Check sheet for the modelled part. Datum: model origin and axes. Units: mm. A direction names the side the tool comes from. Coordinates: 2 decimals unless noted, no trailing zeros. Loops run counter-clockwise (first coordinate to the right, second up) from the corner with the lowest first, then second, coordinate; pieces in that order, holes last. Notation, with made-up numbers: (-35, 82.5) - (-14, 82.5) arc R22 cw to (-14, 91.5) - close; hole circle Ø3 at (79, -30). An arc over 180 degrees is marked (long way). Write each question's results on one line, items separated by ' | '. Start each with the question number.
1. Cross-section at A-A (z = 0). Record the cut outline in (x, y).
2. Draft check along Z on faces 1 (the face through (-27.1, 31.1, -15.4)), 2 (the face through (27.937, 51.549, 15.191)), 3 (the face through (30.092, 33.799, -20.509)). Enter one of: released by +Z, released by -Z, zero draft, split by the parting line, or undercut.
3. Cross-section at B-B (y = 36.75). Record the cut outline in (x, z).
4. Thickness scan on line 1 (Z direction, x = 0, y = 51.45); line 2 (Z direction, x = 0, y = 53.75); line 3 (X direction, y = 52, z = 16). Record the ranges inside material, lowest first. Write a range as [from, to].
5. Gauge pin test, flat ends, axial feed: P1, Ø1, axis at y = 32.5, z = 36.5, coming from the -X side; P2, Ø1.8, axis at x = 25.49, z = 13.83, coming from the -Y side; P3, Ø12, axis at y = 35.5, z = -0.5, coming from the -X side; P4, Ø4, axis at x = -8.5, y = 50.5, coming from the +Z side. Record the tip position at first contact, or that the pin passes through.
6. Tool access check on faces 4 (the face through (32.8, 33.8, -15.8)), 5 (the face through (31, 34.1, -19)), 6 (the face through (-29.95, 32.086, -20.756)). Record the directions out of +Z, -Z, +X, -X, +Y, -Y that give a thin tool (end or side, any length) a straight path to the whole face; none if there is none.
```python
from build123d import *

# Parameters (mm, degrees)
SKETCH1_R                = 35
SKETCH1_R_2              = 2.6
SKETCH1_R_3              = 11
BOSS_EXTRUDE1_DEPTH      = 50
SKETCH2_R                = 31
CUT_EXTRUDE1_DEPTH       = 45
SKETCH3_R                = 26.05
SKETCH3_R_2              = 23.55
BOSS_EXTRUDE2_DEPTH      = 7.5
BOSS_EXTRUDE3_START      = -8
SKETCH5_R                = 23.55
SKETCH5_R_2              = 20.75
BOSS_EXTRUDE3_DEPTH      = 2
SKETCH7_R                = 35
SKETCH7_R_2              = 25.333529331
BOSS_EXTRUDE4_DEPTH      = 7.5
SKETCH9_R                = 31
SKETCH9_R_2              = 26.05
CUT_EXTRUDE2_DEPTH       = 10
FILLET1_R                = 3
SKETCH11_R               = 26.883478625
CUT_EXTRUDE4_DEPTH       = 404
SKETCH12_R               = 1.5
CUT_EXTRUDE5_DEPTH       = 7
CUT_EXTRUDE6_DEPTH       = 7
CIRPATTERN1_COUNT        = 3
SKETCH15_R               = 26.05
SKETCH15_R_2             = 20.75
BOSS_EXTRUDE5_DEPTH      = 3
SKETCH10_W               = 144.751988019
SKETCH10_H               = 48.841098946
CUT_EXTRUDE7_DEPTH       = 93
CUT_EXTRUDE7_DEPTH_BACK  = 113
SKETCH16_R               = 1.5
BOSS_EXTRUDE6_DEPTH      = 3
FILLET3_R                = 1
CIRPATTERN7_COUNT        = 3
FILLET3_OF_CIRPATTERN7_R = 1


with BuildPart() as part:
    # Sketch1 → Boss-Extrude1 (new body)
    with BuildSketch(Plane(origin=(0, 0, 0), x_dir=(1, 0, 0), z_dir=(0, 1, 0))):
        Circle(SKETCH1_R)
        with Locations((-8.350111435, 15.379390073)):
            Circle(SKETCH1_R_2, mode=Mode.SUBTRACT)
        with Locations((-9.143886781, -14.921103663)):
            Circle(SKETCH1_R_2, mode=Mode.SUBTRACT)
        with Locations((17.493998216, -0.45828641)):
            Circle(SKETCH1_R_2, mode=Mode.SUBTRACT)
        Circle(SKETCH1_R_3, mode=Mode.SUBTRACT)
    extrude(amount=BOSS_EXTRUDE1_DEPTH)

    # Sketch2 → Cut-Extrude1 (cut)
    with BuildSketch(Plane.XZ):
        Circle(SKETCH2_R)
    extrude(amount=-CUT_EXTRUDE1_DEPTH, mode=Mode.SUBTRACT)

    # Sketch3 → Boss-Extrude2 (add)
    with BuildSketch(Plane(origin=(0, 50, 0), x_dir=(1, 0, 0), z_dir=(0, 1, 0))):
        with Locations((0, 0.716470669)):
            Circle(SKETCH3_R)
        Circle(SKETCH3_R_2, mode=Mode.SUBTRACT)
    extrude(amount=BOSS_EXTRUDE2_DEPTH)

    # Sketch5 → Boss-Extrude3 (add)
    with BuildSketch(Plane(origin=(0, 57.5, 0), x_dir=(1, 0, 0), z_dir=(0, 1, 0)).offset(BOSS_EXTRUDE3_START)):
        Circle(SKETCH5_R)
        Circle(SKETCH5_R_2, mode=Mode.SUBTRACT)
    extrude(amount=BOSS_EXTRUDE3_DEPTH)

    # Sketch7 → Boss-Extrude4 (add)
    with BuildSketch(Plane(origin=(0, 50, 0), x_dir=(1, 0, 0), z_dir=(0, 1, 0))):
        Circle(SKETCH7_R)
        Circle(SKETCH7_R_2, mode=Mode.SUBTRACT)
    extrude(amount=BOSS_EXTRUDE4_DEPTH)

    # Sketch9 → Cut-Extrude2 (cut)
    with BuildSketch(Plane.XZ.offset(-45)):
        Circle(SKETCH9_R)
        Circle(SKETCH9_R_2, mode=Mode.SUBTRACT)
    extrude(amount=-CUT_EXTRUDE2_DEPTH, mode=Mode.SUBTRACT)

    # Fillet1
    fillet1_edges = [part.edges().sort_by_distance(p)[0] for p in [
        (-23.55, 57.5, 0),
        (-35, 57.5, 0),
    ]]
    fillet(fillet1_edges, radius=FILLET1_R)

    # Sketch11 → Cut-Extrude4 (cut)
    with BuildSketch(Plane(origin=(0, 50, 0), x_dir=(1, 0, 0), z_dir=(0, 1, 0))):
        Circle(SKETCH11_R)
    extrude(amount=-CUT_EXTRUDE4_DEPTH, mode=Mode.SUBTRACT)

    # Sketch12 → Cut-Extrude5 (cut)
    with BuildSketch(Plane(origin=(0, 57.5, 0), x_dir=(1, 0, 0), z_dir=(0, 1, 0))):
        with Locations((-0.762925985, 28.989962814)):
            Circle(SKETCH12_R)
    cut_extrude5 = extrude(amount=-CUT_EXTRUDE5_DEPTH, mode=Mode.SUBTRACT)

    # Sketch13 → Cut-Extrude6 (cut)
    with BuildSketch(Plane.XZ.offset(-55)):
        Polygon((-3.995941284, -28.959215343), (-2.406061725, -31.774462459), (0.826953574, -31.805209929), (2.470089315, -29.020710284), (0.880209755, -26.205463169), (-2.352805544, -26.174715698), align=None)
    cut_extrude6 = extrude(amount=CUT_EXTRUDE6_DEPTH, mode=Mode.SUBTRACT)

    # CirPattern1: Cut-Extrude5, Cut-Extrude6 ×3 about axis
    cirpattern1_axis = Axis((0, 0, 0), (0, 1, 0))
    for i in range(1, CIRPATTERN1_COUNT):
        add(cut_extrude5.rotate(cirpattern1_axis, i * 360 / CIRPATTERN1_COUNT), mode=Mode.SUBTRACT)
        add(cut_extrude6.rotate(cirpattern1_axis, i * 360 / CIRPATTERN1_COUNT), mode=Mode.SUBTRACT)

    # Sketch15 → Boss-Extrude5 (add)
    with BuildSketch(Plane.XZ.offset(-50)):
        Circle(SKETCH15_R)
        Circle(SKETCH15_R_2, mode=Mode.SUBTRACT)
    extrude(amount=-BOSS_EXTRUDE5_DEPTH)

    # Sketch10 → Cut-Extrude7 (cut, two sides)
    with BuildSketch(Plane(origin=(0, 0, 0), x_dir=(0, 0, -1), z_dir=(1, 0, 0))) as cut_extrude7_sk:
        with Locations((-1.20572645, 6.679450527)):
            Rectangle(SKETCH10_W, SKETCH10_H)
    extrude(amount=CUT_EXTRUDE7_DEPTH, mode=Mode.SUBTRACT)
    extrude(cut_extrude7_sk.sketch, amount=-CUT_EXTRUDE7_DEPTH_BACK, mode=Mode.SUBTRACT)

    # Sketch16 → Boss-Extrude6 (add)
    with BuildSketch(Plane.XZ.offset(-31.1)):
        with BuildLine():
            Line((-3, 34.871191548), (-3, 37.8))
            ThreePointArc((-3, 37.8), (0, 40.8), (3, 37.8))
            Line((3, 37.8), (3, 34.871191548))
            Line((3, 34.871191548), (-3, 34.871191548))
        make_face()
        with Locations((0, 37.8)):
            Circle(SKETCH16_R, mode=Mode.SUBTRACT)
    boss_extrude6 = extrude(amount=-BOSS_EXTRUDE6_DEPTH)

    # Fillet3
    fillet3_edges = [part.edges().sort_by_distance(p)[0] for p in [
        (-3, 34.1, 36.335595774),
        (0, 34.1, 40.8),
        (3, 34.1, 36.335595774),
    ]]
    fillet(fillet3_edges, radius=FILLET3_R)

    # CirPattern7: Boss-Extrude6 ×3 about axis
    cirpattern7_axis = Axis((0, 0, 0), (0, 1, 0))
    for i in range(1, CIRPATTERN7_COUNT):
        add(boss_extrude6.rotate(cirpattern7_axis, i * 360 / CIRPATTERN7_COUNT))

    # Fillet3 of CirPattern7
    fillet3_of_cirpattern7_edges = [part.edges().sort_by_distance(p)[0] for p in [
        (32.967549002, 34.1, -15.569721676),
        (35.333836474, 34.1, -20.4),
        (29.967549002, 34.1, -20.765874098),
        (-29.967549002, 34.1, -20.765874098),
        (-35.333836474, 34.1, -20.4),
        (-32.967549002, 34.1, -15.569721676),
    ]]
    fillet(fillet3_of_cirpattern7_edges, radius=FILLET3_OF_CIRPATTERN7_R)


solid = part.part
```
Established:
1) outline: (-35, 31.1) - (-31, 31.1) - (-31, 55) - (-26.05, 55) - (-26.05, 50) - (-20.75, 50) - (-20.75, 53) - (-23.55, 53) - (-23.55, 54.5) arc R3 ccw to (-26.55, 57.5) - (-32, 57.5) arc R3 ccw to (-35, 54.5) - close; (20.75, 50) - (26.05, 50) - (26.05, 55) - (31, 55) - (31, 31.1) - (35, 31.1) - (35, 54.5) arc R3 ccw to (32, 57.5) - (26.55, 57.5) arc R3 ccw to (23.55, 54.5) - (23.55, 53) - (20.75, 53) - close
2) face 1: zero draft | face 2: undercut | face 3: released by -Z
3) outline: circle Ø70 at (0, 0); hole circle Ø62 at (0, 0)
4) line 1: [-35, -31.8], [-26.05, -20.75], [20.75, 26.05], [31, 35] | line 2: [-35, -31.8], [-26.05, -23.55], [23.55, 26.05], [31, 35] | line 3: [-31.13, -27.48], [-20.56, -13.21], [13.21, 20.56], [27.48, 31.13]
5) P1: x = -3 | P2: through | P3: x = -35 | P4: z = 34.39
6) face 4: +X, +Y | face 5: -Z, +X, +Y | face 6: -Z, +Y, -Y
